from build123d import *

# Parameters (mm, degrees)
F1_W     = 190
F1_H     = 55
F1_R     = 3
F1_W_2   = 120
F1_H_2   = 20
F2_DEPTH = 6
F7_DEPTH = 5
F8_DEPTH = 10


with BuildPart() as f2:
    # F1 (on Front) → F2 (new body)
    with BuildSketch(Plane.XZ):
        with Locations((75, 17.5)):
            Rectangle(F1_W, F1_H)
        with Locations((-10, 35)):
            Circle(F1_R, mode=Mode.SUBTRACT)
        with Locations((75, 17.5)):
            Rectangle(F1_W_2, F1_H_2, mode=Mode.SUBTRACT)
        with Locations((160, 35)):
            Circle(F1_R, mode=Mode.SUBTRACT)
    extrude(amount=F2_DEPTH)

    # F6 (on offset) → F7 (join, symmetric)
    with BuildSketch(Plane.YZ.offset(10)):
        with BuildLine():
            Line((-38.885744, 26.227702), (-37.657016, 27.088066))
            Line((-37.657016, 27.088066), (-31.921252, 18.896546))
            Line((-31.921252, 18.896546), (-28.711814, 21.143818))
            Line((-28.711814, 21.143818), (-39.086786, 35.960815))
            Line((-39.086786, 35.960815), (-40.183468, 37.527037))
            Line((-40.183468, 37.527037), (-43.460076, 35.232732))
            Line((-43.460076, 35.232732), (-42.582241, 34.087168))
            ThreePointArc((-42.582241, 34.087168), (-43.698463, 31.404123), (-42.907039, 28.607995))
            Line((-42.907039, 28.607995), (-40.612733, 25.331387))
            Line((-40.612733, 25.331387), (-39.183706, 24.517514))
            Line((-39.183706, 24.517514), (-38.364554, 25.09109))
            Line((-38.364554, 25.09109), (-39.070053, 26.098647))
            Line((-39.070053, 26.098647), (-38.885744, 26.227702))
        make_face()
        with BuildLine():
            Line((-39.086786, 35.960815), (-28.711814, 21.143818))
            ThreePointArc((-28.711814, 21.143818), (-16.759457, 24.582262), (-4.374549, 25.720592))
            Line((-4.374549, 25.720592), (-4.374549, 35.960815))
            Line((-4.374549, 35.960815), (-39.086786, 35.960815))
        make_face()
        with BuildLine():
            ThreePointArc((-17.949438, -7.035153), (-15.59262, -8.73518), (-12.689612, -8.60393))
            Line((-12.689612, -8.60393), (-17.581842, -1.582256))
            Line((-17.581842, -1.582256), (-17.58209, -1.581899))
            Line((-17.58209, -1.581899), (-18.995128, -2.571318))
            Line((-18.995128, -2.571318), (-19.700627, -1.563761))
            Line((-19.700627, -1.563761), (-20.519779, -2.137338))
            Line((-20.519779, -2.137338), (-20.243744, -3.758545))
            Line((-20.243744, -3.758545), (-17.949438, -7.035153))
        make_face()
        Polygon((-17.581842, -1.582256), (-12.689612, -8.60393), (-12.027587, -9.800477), (-8.750979, -7.506171), (-20.222507, 8.876869), (-23.364775, 6.67663), (-17.58209, -1.581899), align=None)
        with BuildLine():
            Line((-20.222507, 8.876869), (-8.750979, -7.506171))
            Line((-8.750979, -7.506171), (-4.07082, -7.506171))
            Line((-4.07082, -7.506171), (-4.07082, 4.745829))
            ThreePointArc((-4.07082, 4.745829), (-11.783832, 8.229962), (-20.222507, 8.876869))
        make_face()
    extrude(amount=F7_DEPTH, both=True)

    # F5 (on offset) → F8 (join)
    with BuildSketch(Plane.YZ.offset(138)):
        with BuildLine():
            Line((-38.940573, 26.327715), (-37.711845, 27.188079))
            Line((-37.711845, 27.188079), (-31.957074, 19.010133))
            Line((-31.957074, 19.010133), (-28.767087, 21.243786))
            Line((-28.767087, 21.243786), (-39.142092, 36.060827))
            Line((-39.142092, 36.060827), (-40.238616, 37.626827))
            Line((-40.238616, 37.626827), (-43.515224, 35.332521))
            Line((-43.515224, 35.332521), (-42.63707, 34.187181))
            ThreePointArc((-42.63707, 34.187181), (-43.753291, 31.504136), (-42.961868, 28.708008))
            Line((-42.961868, 28.708008), (-40.667562, 25.4314))
            Line((-40.667562, 25.4314), (-39.238535, 24.617526))
            Line((-39.238535, 24.617526), (-38.419383, 25.191103))
            Line((-38.419383, 25.191103), (-39.124882, 26.19866))
            Line((-39.124882, 26.19866), (-38.940573, 26.327715))
        make_face()
        with BuildLine():
            Line((-39.142092, 36.060827), (-28.767087, 21.243786))
            ThreePointArc((-28.767087, 21.243786), (-16.81473, 24.682229), (-4.429822, 25.820559))
            Line((-4.429822, 25.820559), (-4.429822, 36.060827))
            Line((-4.429822, 36.060827), (-39.142092, 36.060827))
        make_face()
        with BuildLine():
            ThreePointArc((-18.004267, -6.93514), (-15.647449, -8.635167), (-12.744441, -8.503917))
            Line((-12.744441, -8.503917), (-17.636671, -1.482243))
            Line((-17.636671, -1.482243), (-17.636919, -1.481886))
            Line((-17.636919, -1.481886), (-19.049957, -2.471305))
            Line((-19.049957, -2.471305), (-19.755456, -1.463748))
            Line((-19.755456, -1.463748), (-20.574608, -2.037325))
            Line((-20.574608, -2.037325), (-20.298572, -3.658532))
            Line((-20.298572, -3.658532), (-18.004267, -6.93514))
        make_face()
        Polygon((-17.636671, -1.482243), (-12.744441, -8.503917), (-12.08271, -9.70067), (-8.806102, -7.406364), (-20.27763, 8.976676), (-23.419604, 6.776643), (-17.636919, -1.481886), align=None)
        with BuildLine():
            Line((-20.27763, 8.976676), (-8.806102, -7.406364))
            Line((-8.806102, -7.406364), (-4.125649, -7.406364))
            Line((-4.125649, -7.406364), (-4.125649, 4.845636))
            ThreePointArc((-4.125649, 4.845636), (-11.838801, 8.329821), (-20.27763, 8.976676))
        make_face()
    extrude(amount=F8_DEPTH)


solid = f2.part
Read the model definition and answer for the solid it produces. Units are mm, in the model's axes. A direction names the side the tool comes from. Coordinates: 2 decimals unless noted, no trailing zeros. Order: outer loops, then holes, each group sorted by start corner. A loop starts at its lowest first (then second) coordinate and runs counter-clockwise, first axis right, second up. Notation, with made-up numbers: (-13, 17.5) - (29, 17.5) arc R29 cw to (29, 43.5) - close; hole circle Ø10 at (21.25, 69.25). An arc over 180 degrees is marked (long way). Use one line per item in the form item = value.
(1) Straight lines are drawn through the part: L1, parallel to X at y = -27, z = 26; L2, parallel to Z at x = -10, y = -2.45; L3, parallel to Y at x = 71.5, z = 37. For each, find the intervals that lie inside material, in ascending order.
Computed values:
L1 = 5 to 15, 138 to 148
L2 = -10 to 32, 38 to 45
L3 = -6 to 0
(2) Section B-B, the plane y = -27 is taken. Give the vertices of the cut face in (x, z), then the cut area to 3 significant figures.
Computed values:
outline = (5, 21.79) - (15, 21.79) - (15, 35.96) - (5, 35.96) - close; (138, 21.91) - (148, 21.91) - (148, 36.06) - (138, 36.06) - close
area = 283 mm²
(3) Given pin 1 Ø2 at (x, y) = (96.5, -8.5) entering from +Z; pin 2 Ø8 at (x, z) = (-10, 35) entering from -Y; pin 3 Ø8.5 at (y, z) = (-16.5, -4.5) entering from +X; pin 4 Ø19 at (y, z) = (-17.5, -3.5) entering from -X, each flat-ended and moving along its own axis, determine where each tip first touches the part or whether it passes through.
Computed values:
pin_1 = through
pin_2 = -6
pin_3 = 148
pin_4 = 5
(4) Section A-A, the plane x = 38 is taken. Give the vertices of the cut face in (y, z).
Computed values:
outline = (-6, -10) - (0, -10) - (0, 7.5) - (-6, 7.5) - close; (-6, 27.5) - (0, 27.5) - (0, 45) - (-6, 45) - close
(5) Which of the six approach directions +Z, -Z, +X, -X, +Y, -Y give full straight-line access (tool end or side, diameter ignored) to faces 4 (the face through (138, -13, 0)), 5 (the face through (143, -22, 36.061)), 6 (the face through (74, -3, 27.5)), 7 (the face through (10.07, -10.41, -8.67))?
Computed values:
face_4 = +Z, -Z, -Y
face_5 = +Z, +X, -X
face_6 = +Y, -Y
face_7 = -Z, +X, -X
(6) For a pull along Z with two mould halves and no side action, classify faces 1 (the face through (10, -22, 35.961)), 2 (the face through (142.93, -43.75, 31.55)), 3 (the face through (5, -25, 30)) as pulls with the +Z half, pulls with the -Z half, needs draft (parallel to the pull), parting line crosses it, or undercut.
Computed values:
face_1 = pulls with the +Z half
face_2 = undercut
face_3 = needs draft
